Geometry: final body of the model. Coordinates: model frame, mm. A direction names the side the tool comes from. Give positions to 0.01 mm unless a question says otherwise; leave off trailing zeros. Loops run counter-clockwise (first coordinate to the right, second up) from the corner with the lowest first, then second, coordinate; pieces in that order, holes last.
from build123d import *

# Parameters (mm, degrees)
SKETCH1_W           = 95.25
SKETCH1_H           = 95.25
SKETCH1_R           = 37.465
BOSS_EXTRUDE1_DEPTH = 3.175
SKETCH2_R           = 2.25
CUT_EXTRUDE1_DEPTH  = 4.175
CIRPATTERN1_COUNT   = 4
FILLET1_R           = 12.7
FILLET2_R           = 3.175


with BuildPart() as part:
    # Sketch1 → Boss-Extrude1 (new body)
    with BuildSketch(Plane(origin=(0, 0, 0), x_dir=(1, 0, 0), z_dir=(0, 1, 0))):
        Rectangle(SKETCH1_W, SKETCH1_H)
        Circle(SKETCH1_R, mode=Mode.SUBTRACT)
    extrude(amount=BOSS_EXTRUDE1_DEPTH)

    # Sketch2 → Cut-Extrude1 (cut, through all)
    with BuildSketch(Plane(origin=(0, 3.175, 0), x_dir=(1, 0, 0), z_dir=(0, 1, 0))):
        with Locations((-34.925, 34.925)):
            Circle(SKETCH2_R)
    cut_extrude1 = extrude(amount=-CUT_EXTRUDE1_DEPTH, mode=Mode.SUBTRACT)

    # CirPattern1: Cut-Extrude1 ×4 about axis
    cirpattern1_axis = Axis((0, 0, 0), (0, 1, 0))
    for i in range(1, CIRPATTERN1_COUNT):
        add(cut_extrude1.rotate(cirpattern1_axis, i * 360 / CIRPATTERN1_COUNT), mode=Mode.SUBTRACT)

    # Fillet1
    fillet1_edges = [part.edges().sort_by_distance(p)[0] for p in [
        (-47.625, 1.5875, -47.625),
        (47.625, 1.5875, -47.625),
        (47.625, 1.5875, 47.625),
        (-47.625, 1.5875, 47.625),
    ]]
    fillet(fillet1_edges, radius=FILLET1_R)

    # Sketch4 → Revolve1 (revolve)
    with BuildSketch(Plane.XY):
        Polygon((37.465, 9.525), (37.465, 3.175), (38.1, 3.175), (38.1, 10.3505), (38.1, 11.1125), (37.465, 12.7), align=None)
    revolve(axis=Axis((0, 0, 0), (0, 1, 0)))

    # Fillet2
    fillet2_edges = [part.edges().sort_by_distance(p)[0] for p in [
        (-38.1, 3.175, 0),
    ]]
    fillet(fillet2_edges, radius=FILLET2_R)


solid = part.part
Item 1: Ray query, probe 1 along Z at (x, y) = (0, 9) (3 decimals); probe 2 along Z at (x, y) = (34.5, 2.25) (1 decimal). Return the intervals inside material, ascending.
Values follow:
probe 1: z = -38.1 to -37.465, 37.465 to 38.1
probe 2: z = -47.6 to -37.1, -32.7 to -14.6, 14.6 to 32.7, 37.1 to 47.6
Item 2: Draft query along X for faces 3 (the face through (-32, 0, -22)), 4 (the face through (47.625, 2, 0)), 5 (the face through (-33.556, 1.61, 36.711)). Return one class per face: +X half, -X half, draft (parallel to the pull), parting line (faces both ways), or undercut.
Values follow:
face 3: draft
face 4: +X half
face 5: undercut
Item 3: Set-up query: faces 1 (the face through (36.711, 1.61, 33.556)), 2 (the face through (42, 3.175, -1)). Return all of +Z, -Z, +X, -X, +Y, -Y with unobstructed straight access to the full face (end or side cutting, diameter ignored); none if empty.
Values follow:
face 1: +Y, -Y
face 2: +Y
Item 4: Section query C-C on y = 1.25. Return loops of the section in (x, z) (3 decimals), plus the area to 3 significant figures.
Values follow:
outline: (-47.625, -34.925) arc R12.7 ccw to (-34.925, -47.625) - (34.925, -47.625) arc R12.7 ccw to (47.625, -34.925) - (47.625, 34.925) arc R12.7 ccw to (34.925, 47.625) - (-34.925, 47.625) arc R12.7 ccw to (-47.625, 34.925) - close; hole circle Ø74.93 at (0, 0); hole circle Ø4.5 at (-34.925, -34.925); hole circle Ø4.5 at (-34.925, 34.925); hole circle Ø4.5 at (34.925, -34.925); hole circle Ø4.5 at (34.925, 34.925)
area: 4,460 mm2
Item 5: Pin query (flat end, axial travel): pin 1 (5 mm diameter, centred on y = 10.5, z = -4.5, fed in from -X); pin 2 (2.5 mm diameter, centred on x = -34.925, z = -34.925, fed in from -Y). Return the tip coordinate at first contact, or that it passes through.
Values follow:
pin 1: stops at x = -38.05
pin 2: passes through
